from build123d import *

# Parameters (mm, degrees)
BOSS_EXTRUDE1_DEPTH = 3.05
CUT_EXTRUDE1_DEPTH  = 67.216349945


with BuildPart() as part:
    # Sketch1 → Boss-Extrude1 (new body)
    with BuildSketch(Plane(origin=(0, 0, 0), x_dir=(1, 0, 0), z_dir=(0, 1, 0))):
        with BuildLine():
            Line((12.05, 5.5), (12.05, 0))
            Line((12.05, 0), (54.05, 0))
            Line((54.05, 0), (54.05, 5.5))
            ThreePointArc((54.05, 5.5), (52.989339828, 8.060660172), (55.55, 7))
            Line((55.55, 7), (66.1, 7))
            Line((66.1, 7), (66.1, 11))
            Line((66.1, 11), (63.05, 11))
            Line((63.05, 11), (63.05, 20))
            Line((63.05, 20), (3.05, 20))
            Line((3.05, 20), (3.05, 11))
            Line((3.05, 11), (0, 11))
            Line((0, 11), (0, 7))
            Line((0, 7), (10.55, 7))
            ThreePointArc((10.55, 7), (12.05, 8.5), (13.55, 7))
            ThreePointArc((13.55, 7), (13.110660172, 5.939339828), (12.05, 5.5))
        make_face()
        with BuildLine():
            Line((3.05, 2), (3.05, 0))
            Line((3.05, 0), (12.05, 0))
            Line((12.05, 0), (12.05, 5.5))
            ThreePointArc((12.05, 5.5), (10.989339828, 5.939339828), (10.55, 7))
            Line((10.55, 7), (0, 7))
            Line((0, 7), (0, 2))
            Line((0, 2), (3.05, 2))
        make_face()
        with BuildLine():
            Line((54.05, 5.5), (54.05, 0))
            Line((54.05, 0), (63.05, 0))
            Line((63.05, 0), (63.05, 2))
            Line((63.05, 2), (66.1, 2))
            Line((66.1, 2), (66.1, 7))
            Line((66.1, 7), (55.55, 7))
            ThreePointArc((55.55, 7), (55.110660172, 5.939339828), (54.05, 5.5))
        make_face()
    extrude(amount=BOSS_EXTRUDE1_DEPTH)

    # Sketch5 → CSK for M3 Flat Head Machine Screw1 (revolve, cut)
    with BuildSketch(Plane(origin=(12.05, 3.05, -7), x_dir=(0, 0, 1), z_dir=(1, 0, 0))):
        Polygon((0, 0), (0, 3.05), (1.6, 3.05), (1.6, 1.55), (3.15, 0), align=None)
    revolve(axis=Axis((12.05, 9.4, -7), (0, -1, 0)), mode=Mode.SUBTRACT)

    # Sketch7 → CSK for M3 Flat Head Machine Screw2 (revolve, cut)
    with BuildSketch(Plane(origin=(54.05, 3.05, -7), x_dir=(0, 0, 1), z_dir=(1, 0, 0))):
        Polygon((0, 0), (0, 3.05), (1.6, 3.05), (1.6, 1.55), (3.15, 0), align=None)
    revolve(axis=Axis((54.05, 9.4, -7), (0, -1, 0)), mode=Mode.SUBTRACT)

    # Sketch8 → Cut-Extrude1 (cut, through all)
    with BuildSketch(Plane.ZY.offset(-3.05)):
        Polygon((-20, 0), (-20, 3.05), (-16.223809523, 0), align=None)
    extrude(amount=-CUT_EXTRUDE1_DEPTH, mode=Mode.SUBTRACT)


solid = part.part
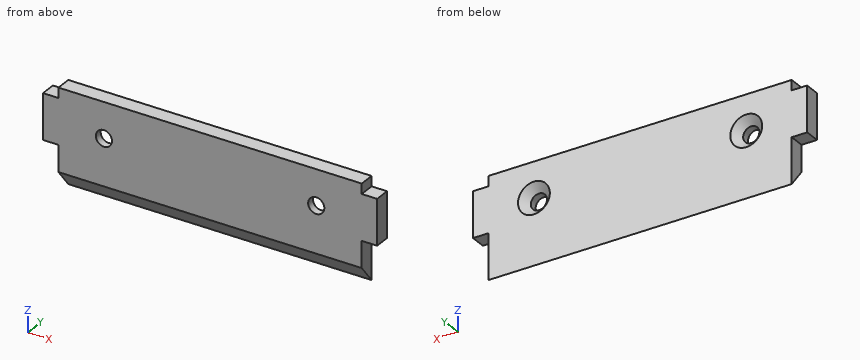
Verification items for the finished model (mm, model axes). Coordinates: 2 decimals unless noted, no trailing zeros. Order: outer loops, then holes, each group sorted by start corner. A loop starts at its lowest first (then second) coordinate and runs counter-clockwise, first axis right, second up.
1. Sectioned sample at D-D, the plane x = 19. Record the cut outline in (y, z).
Results found:
outline: (0, -16.22) - (3.05, -20) - (3.05, 0) - (0, 0) - close
2. Sectioned sample at B-B, the plane z = -7. Record the cut outline in (x, y), and give its area (3 significant figures).
Results found:
outline: (0, 0) - (10.45, 0) - (10.45, 1.5) - (8.9, 3.05) - (0, 3.05) - close; (13.65, 0) - (52.45, 0) - (52.45, 1.5) - (50.9, 3.05) - (15.2, 3.05) - (13.65, 1.5) - close; (55.65, 0) - (66.1, 0) - (66.1, 3.05) - (57.2, 3.05) - (55.65, 1.5) - close
area: 177 mm2
3. Sectioned sample at A-A, the plane x = 12.05. Record the cut outline in (y, z), and give its area (3 significant figures).
Results found:
outline: (0, -16.22) - (3.05, -20) - (3.05, -10.15) - (1.5, -8.6) - (0, -8.6) - close; (0, -5.4) - (1.5, -5.4) - (3.05, -3.85) - (3.05, 0) - (0, 0) - close
area: 43.1 mm2
4. Scan lines: line 1 (X direction, y = 0.35, z = -7); line 2 (X direction, y = 2.15, z = -9); line 3 (X direction, y = 0.4, z = -1.5). Record each from-to range of solid material in increasing order.
Results found:
line 1: x = 0 to 10.45, 13.65 to 52.45, 55.65 to 66.1
line 2: x = 0 to 11.02, 13.08 to 53.02, 55.08 to 66.1
line 3: x = 3.05 to 63.05
5. Go/stop test with flat-tipped pins: pin 1 Ø6 at (x, z) = (29, -14) entering from -Y; pin 2 Ø4 at (x, z) = (54.05, -7) entering from +Y; pin 3 Ø1.5 at (y, z) = (1.5, -15.5) entering from +X; pin 4 Ø1.5 at (x, y) = (65, 1.5) entering from +Z. Record where each tip stops, or that it passes through.
Results found:
pin 1: stops at y = 0
pin 2: stops at y = 1.9
pin 3: stops at x = 63.05
pin 4: stops at z = -2
6. Sectioned sample at C-C, the plane y = 0.55. Record the cut outline in (x, z), and give its area (3 significant figures).
Results found:
outline: (0, -11) - (3.05, -11) - (3.05, -16.9) - (63.05, -16.9) - (63.05, -11) - (66.1, -11) - (66.1, -2) - (63.05, -2) - (63.05, 0) - (3.05, 0) - (3.05, -2) - (0, -2) - close; hole circle Ø3.2 at (12.05, -7); hole circle Ø3.2 at (54.05, -7)
area: 1,050 mm2
